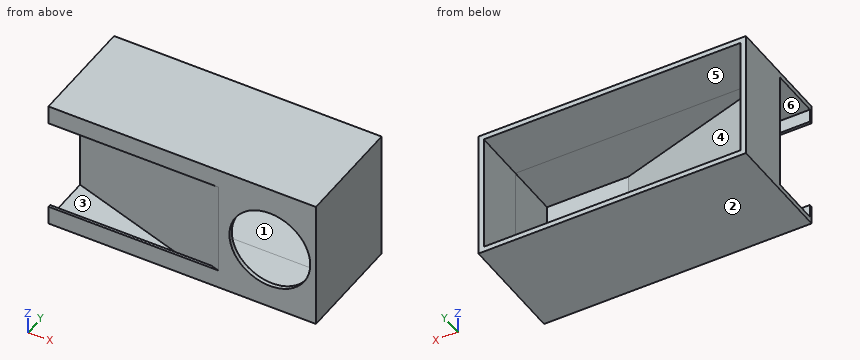
```python
from build123d import *

# Parameters (mm, degrees)
SKETCH1_W            = 200.21
SKETCH1_H            = 97.58
BOSS_EXTRUDE1_DEPTH  = 43
SKETCH2_R            = 30.26
CUT_EXTRUDE1_DEPTH   = 43
SKETCH3_W            = 61.02
SKETCH3_H            = 89.58
CUT_EXTRUDE4_DEPTH   = 40
SKETCH6_W            = 131.19
SKETCH6_H            = 89.58
CUT_EXTRUDE6_DEPTH   = 40
BOSS_EXTRUDE2_DEPTH  = 92
SKETCH10_W           = 200.21
SKETCH10_H           = 4.004947158
BOSS_EXTRUDE3_DEPTH  = 40
SKETCH11_W           = 3.997887423
SKETCH11_H           = 93.575052842
BOSS_EXTRUDE4_DEPTH  = 40
SKETCH14_W           = 198.22617176
SKETCH14_H           = 3.997974015
BOSS_EXTRUDE8_DEPTH  = 40
SKETCH15_W           = 4.000744024
SKETCH15_H           = 90.67582921
BOSS_EXTRUDE9_DEPTH  = 40
CUT_EXTRUDE7_DEPTH   = 93.53
SKETCH17_W           = 133.33152703
SKETCH17_H           = 4
BOSS_EXTRUDE10_DEPTH = 45
SKETCH18_W           = 19.990768927
SKETCH18_H           = 67.482432085
CUT_EXTRUDE8_DEPTH   = 45
SKETCH19_W           = 130.204698474
SKETCH19_H           = 63.111611145
CUT_EXTRUDE9_DEPTH   = 45
BOSS_EXTRUDE11_DEPTH = 10
BOSS_EXTRUDE12_DEPTH = 10


with BuildPart() as part:
    # Sketch1 → Boss-Extrude1 (new body)
    with BuildSketch(Plane(origin=(0, 0, 0), x_dir=(1, 0, 0), z_dir=(0, 1, 0))):
        with Locations((100.105, 48.79)):
            Rectangle(SKETCH1_W, SKETCH1_H)
    extrude(amount=BOSS_EXTRUDE1_DEPTH)

    # Sketch2 → Cut-Extrude1 (cut)
    with BuildSketch(Plane(origin=(0, 43, 0), x_dir=(1, 0, 0), z_dir=(0, 1, 0))):
        with Locations(Location((165.7, 49.98, 0), (0, 0, 270))):
            Circle(SKETCH2_R)
    extrude(amount=-CUT_EXTRUDE1_DEPTH, mode=Mode.SUBTRACT)

    # Sketch3 → Cut-Extrude4 (cut)
    with BuildSketch(Plane(origin=(0, 43, 0), x_dir=(1, 0, 0), z_dir=(0, 1, 0))):
        with Locations((165.7, 48.79)):
            Rectangle(SKETCH3_W, SKETCH3_H)
    extrude(amount=-CUT_EXTRUDE4_DEPTH, mode=Mode.SUBTRACT)

    # Sketch6 → Cut-Extrude6 (cut)
    with BuildSketch(Plane(origin=(0, 43, 0), x_dir=(1, 0, 0), z_dir=(0, 1, 0))):
        with Locations((69.595, 48.79)):
            Rectangle(SKETCH6_W, SKETCH6_H)
    extrude(amount=-CUT_EXTRUDE6_DEPTH, mode=Mode.SUBTRACT)

    # Sketch9 → Boss-Extrude2 (add)
    with BuildSketch(Plane.XY.offset(-93.58)):
        Polygon((4, 3), (135.19, 3), (4, 43), align=None)
    extrude(amount=BOSS_EXTRUDE2_DEPTH)

    # Sketch10 → Boss-Extrude3 (add)
    with BuildSketch(Plane(origin=(0, 43, 0), x_dir=(1, 0, 0), z_dir=(0, 1, 0))):
        with Locations((100.105, 2.002473579)):
            Rectangle(SKETCH10_W, SKETCH10_H)
    extrude(amount=BOSS_EXTRUDE3_DEPTH)

    # Sketch11 → Boss-Extrude4 (add)
    with BuildSketch(Plane(origin=(0, 43, 0), x_dir=(1, 0, 0), z_dir=(0, 1, 0))):
        with Locations((1.998943712, 50.792473579)):
            Rectangle(SKETCH11_W, SKETCH11_H)
    extrude(amount=BOSS_EXTRUDE4_DEPTH)

    # Sketch14 → Boss-Extrude8 (add)
    with BuildSketch(Plane(origin=(0, 43, 0), x_dir=(1, 0, 0), z_dir=(0, 1, 0))):
        with Locations((101.09691412, 95.581012993)):
            Rectangle(SKETCH14_W, SKETCH14_H)
    extrude(amount=BOSS_EXTRUDE8_DEPTH)

    # Sketch15 → Boss-Extrude9 (add)
    with BuildSketch(Plane(origin=(0, 43, 0), x_dir=(1, 0, 0), z_dir=(0, 1, 0))):
        with Locations((198.209627988, 49.342861763)):
            Rectangle(SKETCH15_W, SKETCH15_H)
    extrude(amount=BOSS_EXTRUDE9_DEPTH)

    # Sketch16 → Cut-Extrude7 (cut)
    with BuildSketch(Plane(origin=(0, 0, -97.58), x_dir=(-1, 0, 0), z_dir=(0, 0, -1))):
        Polygon((0, 0), (-127.19, 0), (0, 40), align=None)
    extrude(amount=-CUT_EXTRUDE7_DEPTH, mode=Mode.SUBTRACT)

    # Sketch17 → Boss-Extrude10 (add)
    with BuildSketch(Plane(origin=(11.44741016, 36.399902458, 0), x_dir=(0.9539379232634473, -0.30000406423883874, 0), z_dir=(-0.30000406423883874, -0.9539379232634474, 0))):
        with Locations((54.665600945, -95.58)):
            Rectangle(SKETCH17_W, SKETCH17_H)
    extrude(amount=BOSS_EXTRUDE10_DEPTH)

    # Sketch18 → Cut-Extrude8 (cut)
    with BuildSketch(Plane(origin=(0, 0, -97.58), x_dir=(-1, 0, 0), z_dir=(0, 0, -1))):
        with Locations((9.995384464, 19.727595476)):
            Rectangle(SKETCH18_W, SKETCH18_H)
    extrude(amount=-CUT_EXTRUDE8_DEPTH, mode=Mode.SUBTRACT)

    # Sketch19 → Cut-Extrude9 (cut)
    with BuildSketch(Plane(origin=(0, 0, -97.58), x_dir=(-1, 0, 0), z_dir=(0, 0, -1))):
        with Locations((-62.087650763, -31.555805573)):
            Rectangle(SKETCH19_W, SKETCH19_H)
    extrude(amount=-CUT_EXTRUDE9_DEPTH, mode=Mode.SUBTRACT)

    # Sketch20 → Boss-Extrude11 (add)
    with BuildSketch(Plane(origin=(0, 0, -4.05), x_dir=(-1, 0, 0), z_dir=(0, 0, -1))):
        Polygon((0, 0), (0, 2), (-120.8305, 2), (-127.19, 0), align=None)
    extrude(amount=BOSS_EXTRUDE11_DEPTH)

    # Sketch21 → Boss-Extrude12 (add)
    with BuildSketch(Plane.XY.offset(-93.58)):
        Polygon((0, 0), (0, 2), (120.8305, 2), (127.19, 0), align=None)
    extrude(amount=BOSS_EXTRUDE12_DEPTH)


solid = part.part
```
For this review, take the finished solid that the model builds, in its own axes (mm). Face numbers are marked on the shaded views. A direction names the side the tool comes from. Coordinates: 2 decimals unless noted, no trailing zeros. Loops run counter-clockwise (first coordinate to the right, second up) from the corner with the lowest first, then second, coordinate; pieces in that order, holes last. Notation, with made-up numbers: (41, 11.5) -> (78, 11.5) arc R30 ccw to (78, 50.5) -> close; hole circle Ø4 at (25.5, 74.25). An arc over 180 degrees is marked (long way). Return JSON: item names as keys, results as strings. Group by question number.
(1) Mouldability with a two-part tool opening along Y and no side actions: class the marked faces 3, 4, 5 and 6 as pulls with the +Y half, pulls with the -Y half, needs draft (parallel to the pull), parting line crosses it, or undercut.
(2) Tool access review of the marked faces 1 and 2: name each direction out of +Z, -Z, +X, -X, +Y, -Y from which nothing blocks a thin tool from reaching the whole face with its end or side.
(3) Consider section C-C, the plane y = 26. Give the boundary of the cut face in (x, z).
(4) For pin 1 Ø0.6 at (x, y) = (76.5, 0.5) entering from +Z; pin 2 Ø2 at (x, z) = (79.5, -19.5) entering from -Y; pin 3 Ø4 at (x, z) = (67, -80) entering from -Y; pin 4 Ø5 at (x, z) = (38, -28) entering from -Y, all flat-tipped, find the tip position at first contact; note any pin that passes through.
(5) To check wall thickness, follow L1, parallel to X at y = 74, z = -28; L2, parallel to Z at x = 165, y = 1; L3, parallel to Z at x = 160.5, y = 4. State the ranges of each line that lie inside material, in increasing order.
Results below:
{
 "1": {"face 3": "undercut", "face 4": "pulls with the +Y half", "face 5": "needs draft", "face 6": "undercut"},
 "2": {"face 1": "+Y", "face 2": "-Z, +X, -X, +Y, -Y"},
 "3": {"outline": "(0, -97.58) -> (200.21, -97.58) -> (200.21, 0) -> (0, 0) -> (0, -4.05) -> (44.52, -4.05) -> (44.52, -93.58) -> (0, -93.58) -> close; hole (59.76, -93.58) -> (196.21, -93.58) -> (196.21, -4) -> (59.76, -4) -> close"},
 "4": {"pin 1": "stops at z = 0", "pin 2": "stops at y = 14.68", "pin 3": "stops at y = 18.3", "pin 4": "stops at y = 27.26"},
 "5": {"L1": "x = 0 to 4, 196.21 to 200.21", "L2": "z = -97.58 to -80.23, -19.73 to 0", "L3": "z = -97.58 to -93.58, -4 to 0"}
}
